from build123d import *

# Parameters (mm, degrees)
SKETCH1_W                = 101.6
SKETCH1_H                = 6.35
BOSS_EXTRUDE1_DEPTH      = 25.4
BOSS_EXTRUDE1_DEPTH_BACK = 24.13
BOSS_EXTRUDE2_DEPTH      = 101.6
SKETCH3_W                = 71.12
SKETCH3_H                = 46.99
CUT_EXTRUDE1_DEPTH       = 1.27
SKETCH4_R                = 6.35
BOSS_EXTRUDE3_DEPTH      = 7.62


with BuildPart() as part:
    # Sketch1 → Boss-Extrude1 (new body, two sides)
    with BuildSketch(Plane.XY) as boss_extrude1_sk:
        with Locations((-50.8, 3.175)):
            Rectangle(SKETCH1_W, SKETCH1_H)
    extrude(amount=BOSS_EXTRUDE1_DEPTH)
    extrude(boss_extrude1_sk.sketch, amount=-BOSS_EXTRUDE1_DEPTH_BACK)

    # Sketch2 → Boss-Extrude2 (add)
    with BuildSketch(Plane(origin=(0, 0, 0), x_dir=(0, 0, -1), z_dir=(1, 0, 0))):
        Polygon((-25.4, 6.35), (3.175, 55.843351826), (6.474556788, 53.938351826), (-21.000590949, 6.35), align=None)
    extrude(amount=-BOSS_EXTRUDE2_DEPTH)

    # Sketch3 → Cut-Extrude1 (cut)
    with BuildSketch(Plane(origin=(0, 12.586022628, 21.799630657), x_dir=(1, 0, 0), z_dir=(0, 0.5, 0.866025404))):
        with Locations((-60.96, 21.374261314)):
            Rectangle(SKETCH3_W, SKETCH3_H)
    extrude(amount=-CUT_EXTRUDE1_DEPTH, mode=Mode.SUBTRACT)

    # Sketch4 → Boss-Extrude3 (add)
    with BuildSketch(Plane(origin=(0, 12.586022628, 21.799630657), x_dir=(1, 0, 0), z_dir=(0, 0.5, 0.866025404))):
        with Locations((-12.7, 24.549261314)):
            Circle(SKETCH4_R)
    extrude(amount=BOSS_EXTRUDE3_DEPTH)


solid = part.part
Work out the finished part from the listing and answer in its coordinate system (mm). A direction names the side the tool comes from. Give positions to 0.01 mm unless a question says otherwise; leave off trailing zeros. Write each loop counter-clockwise with the first axis right and the second up, starting at its lowest first coordinate (ties: lowest second). Pieces come first, ordered by that corner, then holes. Notation, with made-up numbers: (-33, 16) - (-23, 16) arc R14 cw to (-23, 41) - close; hole circle Ø6 at (35.5, -33.5). An arc over 180 degrees is marked (long way). One line per item, written item: value. Start each with the question number.
1. Find section D-D (z = -19.5). Write down the section's boundary in (x, y), then the cut area to 3 significant figures.
2. Find section C-C (y = 44.5). Write down the section's boundary in (x, z).
3. For a pull along X with two mould halves and no side action, classify faces 3 (the flat face through (-101.6, 5, 4)), 4 (the flat face through (-61.458, 30.747, 9.848)), 5 (the flat face through (-52, 0, 1)), 6 (the flat face through (-25.4, 30, 11)) as +X half, -X half, draft (parallel to the pull), parting line (faces both ways), or undercut.
4. For faces 1 (the flat face through (-50.09, 30.48, 7.07)), 2 (the flat face through (-52, 3, -24.13)), determine the directions among +Z, -Z, +X, -X, +Y, -Y from which every point of the face is accessible in a straight line to the end or side of a thin tool.
5. Given pin 1 (5 mm diameter, centred on x = -23.5, y = 36.5, fed in from +Z); pin 2 (12.5 mm diameter, centred on y = 22.5, z = 16.5, fed in from +X); pin 3 (5 mm diameter, centred on x = -20.5, y = 23.5, fed in from -Z); pin 4 (5 mm diameter, centred on x = -61, y = 16, fed in from +Z), each flat-ended and moving along its own axis, determine where each tip first touches the part or whether it passes through.
6. Consider probe 1 along X at (y, z) = (22, 15); probe 2 along Y at (x, z) = (-20, -21.5); probe 3 along Y at (x, z) = (-27.5, 9). Determine where each line is inside the solid, lowest interval first.
7. Find section A-A (z = -5). Write down the section's boundary in (x, y), then the cut area to 3 significant figures.
8. Find section B-B (x = -92.5). Write down the section's boundary in (y, z) (3 decimals).
Geometry results:
1. outline: (-101.6, 0) - (0, 0) - (0, 6.35) - (-101.6, 6.35) - close
1. area: 645 mm2
2. outline: (-101.6, -1.03) - (0, -1.03) - (0, 3.37) - (-25.4, 3.37) - (-25.4, 1.91) - (-96.52, 1.91) - (-96.52, 3.37) - (-101.6, 3.37) - close
3. face 3: -X half
3. face 4: undercut
3. face 5: draft
3. face 6: undercut
4. face 1: -Z, +X, -X
4. face 2: -Z, +X, -X, +Y, -Y
5. pin 1: z = 9.44
5. pin 2: x = 0
5. pin 3: z = 9.66
5. pin 4: z = 19.81
6. probe 1: -101.6 to -96.52, -25.4 to 0
6. probe 2: 0 to 6.35
6. probe 3: 0 to 6.35, 27.14 to 32.22
7. outline: (-101.6, 0) - (0, 0) - (0, 6.35) - (-101.6, 6.35) - close; (-101.6, 51.38) - (0, 51.38) - (0, 54.79) - (-101.6, 54.79) - close
7. area: 991 mm2
8. outline: (0, -24.13) - (6.35, -24.13) - (6.35, 21.001) - (53.938, -6.475) - (55.843, -3.175) - (51.444, -0.635) - (50.809, -1.735) - (10.114, 21.76) - (10.749, 22.86) - (6.35, 25.4) - (0, 25.4) - close
